Here's the drawing with two shaded views (mm, measured from the low corner). I have some questions. A direction names the side the tool comes from. Give positions to 0.01 mm unless a question says otherwise; leave off trailing zeros. Loops run counter-clockwise (first coordinate to the right, second up) from the corner with the lowest first, then second, coordinate; pieces in that order, holes last. Notation, with made-up numbers: (-22, 47.5) -> (26, 47.5) arc R31 cw to (26, 72.5) -> close; hole circle Ø7 at (-21.75, 37). An arc over 180 degrees is marked (long way). Put each result on its own line as item: value.
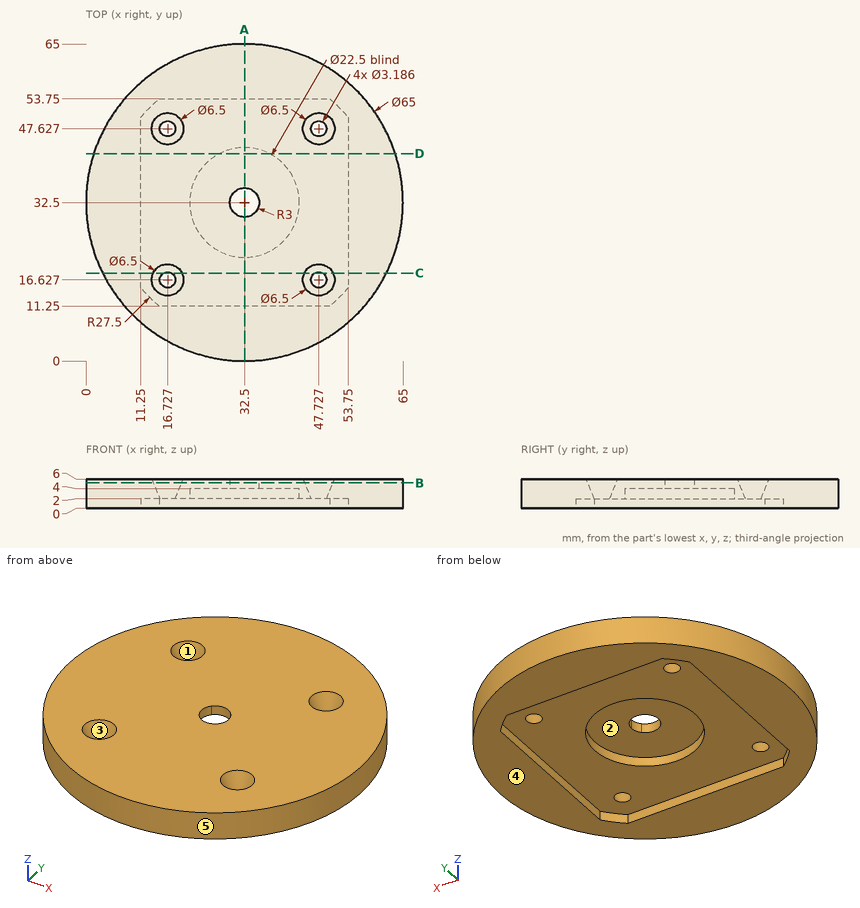
1. If we section it at C-C (y = 18): Count the separate pieces of the cut face and the enclosed holes in it, then the cut area to 3 significant figures.
Recorded:
separate pieces: 3
enclosed holes: 0
area: 233 mm^2
2. I'm going to push flat-ended pins straight in: pin 1 (7 mm diameter, centred on x = 33, y = 37.5, fed in from -Z); pin 2 (20 mm diameter, centred on x = 32.5, y = 32.5, fed in from +Z); pin 3 (1 mm diameter, centred on y = 39.5, z = 1, fed in from +X); pin 4 (1.6 mm diameter, centred on y = 30, z = 0.5, fed in from -X). Where does each tip first touch, or does it pass through?
Recorded:
pin 1: stops at z = 4
pin 2: stops at z = 6
pin 3: stops at x = 64.34
pin 4: stops at x = 0.04
3. I need wall thicknesses on line 1 (Y direction, x = 32.5, z = 2.55); line 2 (Y direction, x = 33, z = 1.9); line 3 (Y direction, x = 46.5, z = 3.1) (1 decimal). Which ranges of each line are inside material? Lowest first, please.
Recorded:
line 1: y = 0 to 21.25, 43.75 to 65
line 2: y = 0 to 11.25, 53.75 to 65
line 3: y = 3.2 to 15, 18.3 to 46, 49.3 to 61.8
4. For the marked faces 1 and 2, which set-ups out of +Z, -Z, +X, -X, +Y, -Y let a thin tool reach every point of the face, with its end or its side?
Recorded:
face 1: +Z
face 2: -Z
5. If we section it at A-A (x = 32.5): List the corners of the cut face in (y, z) for me.
Recorded:
outline: (0, 0) -> (11.25, 0) -> (11.25, 2) -> (21.25, 2) -> (21.25, 4) -> (29.5, 4) -> (29.5, 6) -> (0, 6) -> close; (35.5, 4) -> (43.75, 4) -> (43.75, 2) -> (53.75, 2) -> (53.75, 0) -> (65, 0) -> (65, 6) -> (35.5, 6) -> close
6. If we section it at D-D (y = 42.5): List the corners of the cut face in (x, z) for me.
Recorded:
outline: (1.58, 0) -> (11.25, 0) -> (11.25, 2) -> (27.35, 2) -> (27.35, 4) -> (37.65, 4) -> (37.65, 2) -> (53.75, 2) -> (53.75, 0) -> (63.42, 0) -> (63.42, 6) -> (1.58, 6) -> close
7. If we section it at B-B (z = 5.2): List the corners of the cut face in (x, y) for me, then the cut area to 3 significant figures.
Recorded:
outline: circle Ø65 at (32.5, 32.5); hole circle Ø5.84 at (16.73, 16.63); hole circle Ø5.84 at (16.73, 47.63); hole circle Ø6 at (32.5, 32.5); hole circle Ø5.84 at (47.73, 16.63); hole circle Ø5.84 at (47.73, 47.63)
area: 3,180 mm^2
8. Thinking about a two-plate mould opening in X: for the marked faces 3, 4 and 5, which applies, pulls with the +X half, pulls with the -X half, needs draft (parallel to the pull), parting line crosses it, or undercut?
Recorded:
face 3: undercut
face 4: needs draft
face 5: parting line crosses it
